from build123d import *

# Parameters (mm, degrees)
SKETCH1_W           = 42
SKETCH1_H           = 12
TAILLIGHTBASE_DEPTH = 2
SKETCH2_R           = 0.65
LEDMOUNTS_DEPTH     = 2
SKETCH3_W           = 7
SKETCH3_H           = 12
MOUNTINGTABS_DEPTH  = 2
SKETCH4_R           = 1.375
MOUNTINGHOLES_DEPTH = 2


with BuildPart() as part:
    # Sketch1 → tailLightBase (new body)
    with BuildSketch(Plane.XY):
        with Locations((21, 6)):
            Rectangle(SKETCH1_W, SKETCH1_H)
    extrude(amount=TAILLIGHTBASE_DEPTH)

    # Sketch2 → ledMounts (cut)
    with BuildSketch(Plane.XY.offset(2)):
        with Locations((3, 10.27)):
            Circle(SKETCH2_R)
        with Locations((3, 7.73)):
            Circle(SKETCH2_R)
        with Locations((9, 10.27)):
            Circle(SKETCH2_R)
        with Locations((9, 7.73)):
            Circle(SKETCH2_R)
        with Locations((15, 10.27)):
            Circle(SKETCH2_R)
        with Locations((15, 7.73)):
            Circle(SKETCH2_R)
        with Locations((21, 10.27)):
            Circle(SKETCH2_R)
        with Locations((21, 7.73)):
            Circle(SKETCH2_R)
        with Locations((27, 10.27)):
            Circle(SKETCH2_R)
        with Locations((27, 7.73)):
            Circle(SKETCH2_R)
        with Locations((33, 10.27)):
            Circle(SKETCH2_R)
        with Locations((33, 7.73)):
            Circle(SKETCH2_R)
        with Locations((39, 10.27)):
            Circle(SKETCH2_R)
        with Locations((39, 7.73)):
            Circle(SKETCH2_R)
        with Locations((39, 4.27)):
            Circle(SKETCH2_R)
        with Locations((39, 1.73)):
            Circle(SKETCH2_R)
        with Locations((33, 1.73)):
            Circle(SKETCH2_R)
        with Locations((33, 4.27)):
            Circle(SKETCH2_R)
        with Locations((27, 4.27)):
            Circle(SKETCH2_R)
        with Locations((27, 1.73)):
            Circle(SKETCH2_R)
        with Locations((21, 4.27)):
            Circle(SKETCH2_R)
        with Locations((21, 1.73)):
            Circle(SKETCH2_R)
        with Locations((15, 4.27)):
            Circle(SKETCH2_R)
        with Locations((15, 1.73)):
            Circle(SKETCH2_R)
        with Locations((9, 1.73)):
            Circle(SKETCH2_R)
        with Locations((9, 4.27)):
            Circle(SKETCH2_R)
        with Locations((3, 1.73)):
            Circle(SKETCH2_R)
        with Locations((3, 4.27)):
            Circle(SKETCH2_R)
    extrude(amount=-LEDMOUNTS_DEPTH, mode=Mode.SUBTRACT)

    # Sketch3 → mountingTabs (add)
    with BuildSketch(Plane.XY.offset(2)):
        with Locations((-3.5, 6)):
            Rectangle(SKETCH3_W, SKETCH3_H)
        with Locations((45.5, 6)):
            Rectangle(SKETCH3_W, SKETCH3_H)
    extrude(amount=-MOUNTINGTABS_DEPTH)

    # Sketch4 → mountingHoles (cut)
    with BuildSketch(Plane.XY.offset(2)):
        with Locations((-3.5, 9)):
            Circle(SKETCH4_R)
        with Locations((45.5, 9)):
            Circle(SKETCH4_R)
        with Locations((-3.5, 3)):
            Circle(SKETCH4_R)
        with Locations((45.5, 3)):
            Circle(SKETCH4_R)
    extrude(amount=-MOUNTINGHOLES_DEPTH, mode=Mode.SUBTRACT)


solid = part.part
Design review of the part built by this model. Coordinates are the model's own, in mm. Round coordinates to 2 decimals unless told otherwise and drop trailing zeros. Order: outer loops, then holes, each group sorted by start corner. A loop starts at its lowest first (then second) coordinate and runs counter-clockwise, first axis right, second up.
1) Consider section C-C (z = 1.55). Count the separate pieces of the cut face and the enclosed holes in it, plus the area to 3 significant figures.
The answers:
separate pieces: 1
enclosed holes: 32
area: 611 mm2
2) Consider section B-B (x = 33). State the section outline as (y, z) points, plus the area to 3 significant figures.
The answers:
outline: (0, 0) - (1.08, 0) - (1.08, 2) - (0, 2) - close; (2.38, 0) - (3.62, 0) - (3.62, 2) - (2.38, 2) - close; (4.92, 0) - (7.08, 0) - (7.08, 2) - (4.92, 2) - close; (8.38, 0) - (9.62, 0) - (9.62, 2) - (8.38, 2) - close; (10.92, 0) - (12, 0) - (12, 2) - (10.92, 2) - close
area: 13.6 mm2
3) For L1, parallel to Y at x = 15, z = 0.6; L2, parallel to Y at x = 45.5, z = 1.2 (3 decimals); L3, parallel to Y at x = 33.5, z = 0.4, list the stretches that pass through material, from the lowest coordinate up.
The answers:
L1: y = 0 to 1.08, 2.38 to 3.62, 4.92 to 7.08, 8.38 to 9.62, 10.92 to 12
L2: y = 0 to 1.625, 4.375 to 7.625, 10.375 to 12
L3: y = 0 to 1.31, 2.15 to 3.85, 4.69 to 7.31, 8.15 to 9.85, 10.69 to 12
4) Draft analysis for pull direction X (two halves, no side actions). For faces 1 (the flat face through (49, 6, 1)), 2 (the cylindrical face through (33.6, 7.48, 1.01)), 3 (the flat face through (-7, 6, 1)), 4 (the flat face through (21, 6, 0)), state which applies: released by +X, released by -X, zero draft, split by the parting line, or undercut.
The answers:
face 1: released by +X
face 2: undercut
face 3: released by -X
face 4: zero draft
5) Consider section A-A (y = 9). State the section outline as (x, z) points (3 decimals), plus the area to 3 significant figures.
The answers:
outline: (-7, 0) - (-4.875, 0) - (-4.875, 2) - (-7, 2) - close; (-2.125, 0) - (44.125, 0) - (44.125, 2) - (-2.125, 2) - close; (46.875, 0) - (49, 0) - (49, 2) - (46.875, 2) - close
area: 101 mm2
